```python
from build123d import *

# Parameters (mm, degrees)
CROQUIS2_W              = 20
CROQUIS2_H              = 9
SALIENTE_EXTRUIR1_DEPTH = 30
CROQUIS3_R              = 2.5
CORTAR_EXTRUIR1_DEPTH   = 30
SALIENTE_EXTRUIR2_REACH = 161.769
CROQUIS4_W              = 20
CROQUIS4_H              = 30
CROQUIS5_W              = 14
CROQUIS5_H              = 24
CORTAR_EXTRUIR2_DEPTH   = 11.010004003
SALIENTE_EXTRUIR3_REACH = 98.487
CORTAR_EXTRUIR3_REACH   = 98.487


with BuildPart() as part:
    # Croquis1 → Revolución1 (revolve)
    with BuildSketch(Plane(origin=(0, 0, 0), x_dir=(0, 0, -1), z_dir=(1, 0, 0))):
        Polygon((28.5, 149.256566287), (28.5, 129.256566287), (31.5, 129.256566287), (31.5, 126.256566287), (16, 123.523498086), (16, 63.6684817), (13, 63.6684817), (13, 126.040796979), (25.5, 128.244884238), (25.5, 149.256566287), align=None)
    revolve(axis=Axis((0, 0, 0), (0, 1, 0)))

    # Croquis4 → Saliente-Extruir2 (add, up to next)
    with BuildSketch(Plane.XY.offset(-16), mode=Mode.PRIVATE) as saliente_extruir2_sk1:
        with Locations((0, 98.6684817)):
            Rectangle(CROQUIS4_W, CROQUIS4_H)
    saliente_extruir2_tool1 = extrude(saliente_extruir2_sk1.sketch, amount=SALIENTE_EXTRUIR2_REACH, mode=Mode.PRIVATE) - part.part


with BuildPart() as body_2:
    # Croquis2 → Saliente-Extruir1 (new body)
    with BuildSketch(Plane(origin=(0, 83.6684817, 0), x_dir=(-1, 0, 0), z_dir=(0, -1, 0))):
        with Locations((0, 20.5)):
            Rectangle(CROQUIS2_W, CROQUIS2_H)
    extrude(amount=-SALIENTE_EXTRUIR1_DEPTH)

    # Croquis3 → Cortar-Extruir1 (cut)
    with BuildSketch(Plane(origin=(10, 0, 0), x_dir=(0, 0, -1), z_dir=(1, 0, 0))):
        with Locations((20.5, 98.6684817)):
            Circle(CROQUIS3_R)
    extrude(amount=-CORTAR_EXTRUIR1_DEPTH, mode=Mode.SUBTRACT)


with BuildPart() as part_1:
    add(part.part)

    add(body_2.part)  # Saliente-Extruir2 merges body 2
    add(saliente_extruir2_tool1.solids().sort_by_distance((0, 98.668482, -16))[0])
    add(saliente_extruir2_tool1.solids().sort_by_distance((0, 98.668482, -16))[1])

    # Croquis5 → Cortar-Extruir2 (cut)
    with BuildSketch(Plane(origin=(0, 0, -12.489995997), x_dir=(-1, 0, 0), z_dir=(0, 0, -1))):
        with Locations((0, 98.6684817)):
            Rectangle(CROQUIS5_W, CROQUIS5_H)
    extrude(amount=CORTAR_EXTRUIR2_DEPTH, mode=Mode.SUBTRACT)

    # Saliente-Extruir3: up to this cone (the profile starts outside it)
    saliente_extruir3_end = Plane(origin=(0, 63.668482, 0), z_dir=(0, 1, 0)).offset(57.033785394) * Cone(5.671e-06, 237.928508939, 41.953214606, align=(Align.CENTER, Align.CENTER, Align.MIN), mode=Mode.PRIVATE)
    # Croquis6 → Saliente-Extruir3 (add, up to the surface)
    with BuildSketch(Plane.XZ.offset(-63.6684817), mode=Mode.PRIVATE) as saliente_extruir3_sk1:
        with BuildLine():
            Line((0, -18.227740962), (0, -16))
            ThreePointArc((0, -16), (-2.273055155, -15.837715121), (-4.5, -15.354152533))
            Line((-4.5, -15.354152533), (-4.5, -18.227740962))
            Line((-4.5, -18.227740962), (0, -18.227740962))
        make_face()
    saliente_extruir3_tool1 = extrude(saliente_extruir3_sk1.sketch, amount=-SALIENTE_EXTRUIR3_REACH, mode=Mode.PRIVATE) - saliente_extruir3_end
    add(saliente_extruir3_tool1.solids().sort_by_distance((-2.348795, 63.668482, -16.999565))[0])
    # Croquis6 → Saliente-Extruir3 (add, up to the surface)
    with BuildSketch(Plane.XZ.offset(-63.6684817), mode=Mode.PRIVATE) as saliente_extruir3_sk2:
        with BuildLine():
            ThreePointArc((4.5, -15.354152533), (2.273055155, -15.837715121), (0, -16))
            Line((0, -16), (0, -18.227740962))
            Line((0, -18.227740962), (4.5, -18.227740962))
            Line((4.5, -18.227740962), (4.5, -15.354152533))
        make_face()
    saliente_extruir3_tool2 = extrude(saliente_extruir3_sk2.sketch, amount=-SALIENTE_EXTRUIR3_REACH, mode=Mode.PRIVATE) - saliente_extruir3_end
    add(saliente_extruir3_tool2.solids().sort_by_distance((2.348795, 63.668482, -16.999565))[0])

    # Cortar-Extruir3: up to this cone (the profile starts outside it)
    cortar_extruir3_end = Plane(origin=(0, 63.668482, 0), z_dir=(0, 1, 0)).offset(60.08006523) * Cone(5.671e-06, 220.65219749, 38.90693477, align=(Align.CENTER, Align.CENTER, Align.MIN), mode=Mode.PRIVATE)
    # Croquis7 → Cortar-Extruir3 (cut, up to the surface)
    with BuildSketch(Plane.XZ.offset(-63.6684817), mode=Mode.PRIVATE) as cortar_extruir3_sk1:
        with BuildLine():
            Line((3.5, -17.227740962), (3.5, -15.354152533))
            Line((3.5, -15.354152533), (3.5, -12.519984026))
            ThreePointArc((3.5, -12.519984026), (0, -13), (-3.5, -12.519984026))
            Line((-3.5, -12.519984026), (-3.5, -15.354152533))
            Line((-3.5, -15.354152533), (-3.5, -17.227740962))
            Line((-3.5, -17.227740962), (3.5, -17.227740962))
        make_face()
    cortar_extruir3_tool1 = extrude(cortar_extruir3_sk1.sketch, amount=-CORTAR_EXTRUIR3_REACH, mode=Mode.PRIVATE) - cortar_extruir3_end
    add(cortar_extruir3_tool1.solids().sort_by_distance((0, 63.668482, -15.032146))[0], mode=Mode.SUBTRACT)


solid = part_1.part
```
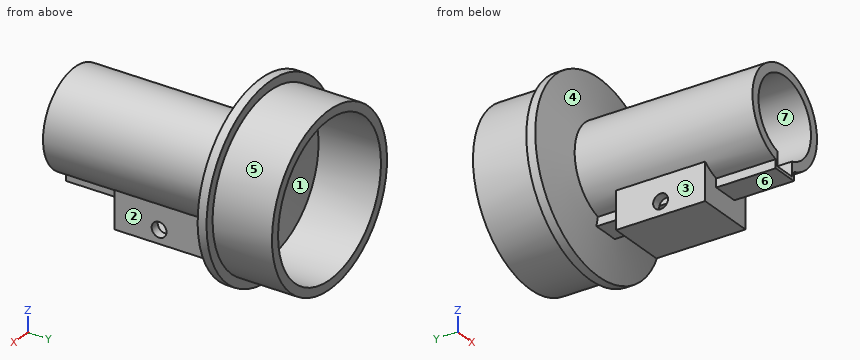
The listing builds one solid part. Answer for the finished solid, in the listing's coordinates (mm). Face numbers are marked on the shaded views. A direction names the side the tool comes from. Round coordinates to 2 decimals unless told otherwise and drop trailing zeros. Loops run counter-clockwise (first coordinate to the right, second up) from the corner with the lowest first, then second, coordinate; pieces in that order, holes last. Notation, with made-up numbers: (36, 14.5) - (79, 14.5) arc R16 cw to (79, 35.5) - close; hole circle Ø4 at (-23, 11.25). An arc over 180 degrees is marked (long way). Return JSON: item names as keys, results as strings. Group by question number.
1. The part is cut by section B-B on y = 73. Determine the outline of the cut face in (x, z), then the cut area to 3 significant figures.
2. Which of the six approach directions +Z, -Z, +X, -X, +Y, -Y give full straight-line access (tool end or side, diameter ignored) to the marked faces 4, 5, 6 and 7?
3. Consider probe 1 along Y at (x, z) = (5.5, -16); probe 2 along Z at (x, y) = (0, 139); probe 3 along Z at (x, y) = (0, 96). Determine where each line is inside the solid, lowest interval first.
4. The part is cut by section C-C on x = 0. Determine the outline of the cut face in (y, z), then the cut area to 3 significant figures.
5. The mould has two halves that part along X. Classify the marked faces 1, 2 and 3: pulls with the +X half, pulls with the -X half, needs draft (parallel to the pull), parting line crosses it, or undercut.
6. The part is cut by section A-A on z = 0. Determine the outline of the cut face in (x, y).
7. Each of these flat-tipped pins is pushed along its axis until it touches: P1, Ø22, axis at x = -1, y = 96, coming from the -Z side; P2, Ø5, axis at x = 20.5, y = 129.5, coming from the -Z side; P3, Ø1, axis at x = 3, y = 115.5, coming from the +Z side. Where does it stop, or does it pass through?
8. The part is cut by section D-D on z = -20.5. State how many separate pieces and enclosed holes the cut face has, then the cut area to 3 significant figures.
Resolved:
{
 "1": {"outline": "(-4.5, -18.23) - (4.5, -18.23) - (4.5, -15.35) arc R16 ccw (long way) to (-4.5, -15.35) - close; hole (-3.5, -17.23) - (3.5, -17.23) - (3.5, -12.52) arc R13 ccw (long way) to (-3.5, -12.52) - close", "area": "265 mm²"},
 "2": {"face 4": "none", "face 5": "+Y", "face 6": "-Z, +X, -X, -Y", "face 7": "+Y, -Y"},
 "3": {"probe 1": "y = 83.67 to 86.67, 110.67 to 113.67, 123.69 to 126.73", "probe 2": "z = -28.5 to -25.5, 25.5 to 28.5", "probe 3": "z = -25 to -23.5, -18.23 to -17.23, 13 to 16"},
 "4": {"outline": "(63.67, -18.23) - (83.67, -18.23) - (83.67, -25) - (113.67, -25) - (113.67, -18.23) - (123.92, -18.23) - (126.26, -31.5) - (129.26, -31.5) - (129.26, -28.5) - (149.26, -28.5) - (149.26, -25.5) - (128.24, -25.5) - (126.79, -17.23) - (63.67, -17.23) - close; (63.67, 13) - (126.04, 13) - (128.24, 25.5) - (149.26, 25.5) - (149.26, 28.5) - (129.26, 28.5) - (129.26, 31.5) - (126.26, 31.5) - (123.52, 16) - (63.67, 16) - close; hole (86.67, -23.5) - (110.67, -23.5) - (110.67, -18.23) - (86.67, -18.23) - close", "area": "541 mm²"},
 "5": {"face 1": "undercut", "face 2": "pulls with the +X half", "face 3": "pulls with the -X half"},
 "6": {"outline": "(-31.5, 126.26) - (-16, 123.52) - (-16, 63.67) - (-13, 63.67) - (-13, 126.04) - (-25.5, 128.24) - (-25.5, 149.26) - (-28.5, 149.26) - (-28.5, 129.26) - (-31.5, 129.26) - close; (13, 63.67) - (16, 63.67) - (16, 123.52) - (31.5, 126.26) - (31.5, 129.26) - (28.5, 129.26) - (28.5, 149.26) - (25.5, 149.26) - (25.5, 128.24) - (13, 126.04) - close"},
 "7": {"P1": "stops at z = -25", "P2": "stops at z = -25.84", "P3": "stops at z = 15.8"},
 "8": {"separate pieces": "3", "enclosed holes": "0", "area": "574 mm²"}
}
